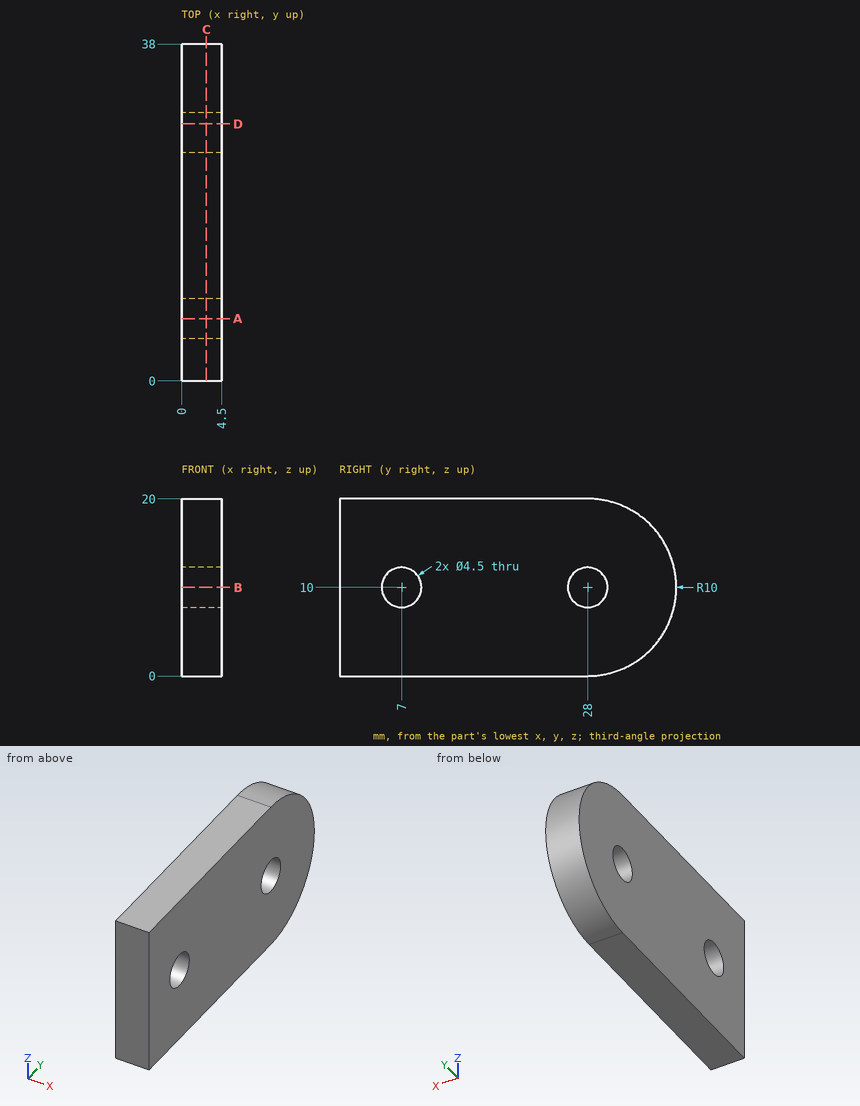
Here's the drawing with two shaded views (mm, measured from the low corner). I have some questions. Coordinates: 2 decimals unless noted, no trailing zeros. Write each loop counter-clockwise with the first axis right and the second up, starting at its lowest first coordinate (ties: lowest second). Pieces come first, ordered by that corner, then holes. Notation, with made-up numbers: (45.5, 36) -> (98.5, 36) arc R29 cw to (98.5, 58) -> close; hole circle Ø8 at (19, 56). An arc over 180 degrees is marked (long way). Use a Markdown table: item, result. Add a question column.
(1) If we section it at C-C, the plane x = 2.8: Write out the boundary of the cut face in (y, z), and give its area (3 significant figures).
(2) Please list where these lines run through material, in increasing order: line 1 (Y direction, x = 1.35, z = 10); line 2 (Z direction, x = 4.15, y = 8.5); line 3 (Y direction, x = 3.65, z = 15.5).
(3) I'm going to push a flat-ended pin straight in: P1, Ø4, axis at y = 7, z = 10, coming from the +X side. Where does the tip first touch, or does it pass through?
(4) If we section it at D-D, the plane y = 29: Write out the boundary of the cut face in (x, z), and give its area (3 significant figures).
(5) If we section it at A-A, the plane y = 7: Write out the boundary of the cut face in (x, z).
(6) If we section it at B-B, the plane z = 10: Write out the boundary of the cut face in (x, y), and give its area (4 significant figures).
Outcome:
| question | item | result |
|---|---|---|
| 1 | outline | (0, 0) -> (28, 0) arc R10 ccw to (28, 20) -> (0, 20) -> close; hole circle Ø4.5 at (7, 10); hole circle Ø4.5 at (28, 10) |
| 1 | area | 685 mm^2 |
| 2 | line 1 | y = 0 to 4.75, 9.25 to 25.75, 30.25 to 38 |
| 2 | line 2 | z = 0 to 8.32, 11.68 to 20 |
| 2 | line 3 | y = 0 to 36.35 |
| 3 | P1 | passes through |
| 4 | outline | (0, 0.05) -> (4.5, 0.05) -> (4.5, 7.98) -> (0, 7.98) -> close; (0, 12.02) -> (4.5, 12.02) -> (4.5, 19.95) -> (0, 19.95) -> close |
| 4 | area | 71.4 mm^2 |
| 5 | outline | (0, 0) -> (4.5, 0) -> (4.5, 7.75) -> (0, 7.75) -> close; (0, 12.25) -> (4.5, 12.25) -> (4.5, 20) -> (0, 20) -> close |
| 6 | outline | (0, 0) -> (4.5, 0) -> (4.5, 4.75) -> (0, 4.75) -> close; (0, 9.25) -> (4.5, 9.25) -> (4.5, 25.75) -> (0, 25.75) -> close; (0, 30.25) -> (4.5, 30.25) -> (4.5, 38) -> (0, 38) -> close |
| 6 | area | 130.5 mm^2 |
